Input: part model. Units: mm. Frame: model coordinates. A direction names the side the tool comes from. Coordinates: 2 decimals unless noted, no trailing zeros. Loops run counter-clockwise (first coordinate to the right, second up) from the corner with the lowest first, then second, coordinate; pieces in that order, holes last. Notation, with made-up numbers: (-15, 63) -> (34, 63) arc R10 ccw to (34, 69) -> close; hole circle Ø8 at (71, 85.25). An arc over 180 degrees is marked (long way). Put each result on its own line as item: value. Start each with the question number.
1) Cut plane A-A (z = 7.5). State how many separate pieces and enclosed holes the cut face has, plus the area to 3 significant figures.
2) Cut plane B-B (x = 19). Return the cut outline in (y, z), plus the area to 3 significant figures.
3) Material intervals for L1, parallel to Y at x = 24.5, z = 7.5; L2, parallel to Y at x = 5, z = 11; L3, parallel to Z at x = 19, y = 16.75, sorted ascending.
4) Cut plane D-D (x = 12.5). Return the cut outline in (y, z), plus the area to 3 significant figures.
5) Set-up query: faces 1 (the flat face through (27, -17, 7)), 2 (the flat face through (11, 14.1, 7.6)). Return all of +Z, -Z, +X, -X, +Y, -Y with unobstructed straight access to the full face (end or side cutting, diameter ignored); none if empty.
6) Contact query for flat-ended pins moving along their axis: P1, Ø1.5, axis at y = 10.5, z = 9.5, coming from the +X side; P2, Ø5.5, axis at x = 19, z = 7.5, coming from the -Y side. Output: stop coordinate, or through.
7) Pull-direction query (Z, two-part tool) for faces 3 (the conical face through (2.29, -18.75, 0.79)), 4 (the cylindrical face through (17.364, -17.128, 7.285)), 5 (the flat face through (13.6, 20.1, 14)), 6 (the flat face through (21, 15.1, 9)); classes: pulls with the +Z half, pulls with the -Z half, needs draft (parallel to the pull), parting line crosses it, or undercut.
Autodesk Inventor part; units mm, degrees
ref_plane "YZ Plane" through (0, 0, 0) normal (1, 0, 0) x (0, 1, 0)
ref_plane "XZ Plane" through (0, 0, 0) normal (0, 1, 0) x (-1, 0, 0)
ref_plane "XY Plane" through (0, 0, 0) normal (0, 0, 1) x (1, 0, 0)
sketch "スケッチ1" plane through (0, 0, 0) normal (0, 0, 1) x (1, 0, 0)
  line L0 (0, 21.1) -> (10, 21.1)
  line L1 (10, 21.1) -> (10, -21.1)
  line L2 (10, -21.1) -> (0, -21.1)
  line L3 (0, -21.1) -> (0, 21.1)
  line L4 (10, 21.1) -> (27, 21.1)
  line L5 (27, 21.1) -> (27, 15.1)
  line L6 (27, 15.1) -> (10, 15.1)
  line L7 (10, 15.1) -> (10, 21.1)
  line L8 (10, -21.1) -> (27, -21.1)
  line L9 (27, -21.1) -> (27, -15.1)
  line L10 (27, -15.1) -> (10, -15.1)
  line L11 (10, -15.1) -> (10, -21.1)
  point P0 (0, 0)
  point P1 (19, 15.1)
  point P2 (10, 15.1)
  dimension "d3" = 8
  dimension "d4" = 10
  dimension "d5" = 30.2
  dimension "d7" = 9
  dimension "d22" = 15.1
  dimension "d25" = 6
  dimension "d26" = 6
extrude "押し出し1" add sketch "スケッチ1" along normal blind 15
sketch "スケッチ2" plane through (0, 21.1, 0) normal (0, 1, 0) x (1, 0, 0)
  line L0 (27, -15) -> (0, -15)
  line L1 (27, 0) -> (27, -15)
  line L2 (27, 0) -> (10, 0)
  line L3 (10, 0) -> (10, -15)
  line L4 (27, -15) -> (10, -15)
  line L5 (27, 0) -> (27, -15)
  point P0 (19, -7.5)
  dimension "d10" = 8
  dimension "d11" = 7.5
hole "穴1" at (19, 21.1, 7.5) direction (0, -1, 0) diameter 3.3 depth 58
sketch "スケッチ3" plane through (0, 21.1, 0) normal (0, 1, 0) x (1, 0, 0)
  circle A0 centre (19, -7.5) radius 1.65
  circle A1 centre (19, -7.5) radius 2.2
  dimension "d19" = 4.4
extrude "押し出し2" cut sketch "スケッチ3" against normal blind 10 contours A0 | A1
fillet "フィレット2" radius 5 6 edges at (27, 18.1, 0) (27, -18.1, 0) (27, -18.1, 15) (27, 18.1, 15) (0, 21.1, 7.5) (0, -21.1, 7.5)
sketch "スケッチ7" plane through (0, 0, 0) normal (0, 0, -1) x (-1, 0, 0)
  circle A0 centre (-5, 0) radius 2.2
  point P0 (0, 0)
  dimension "d55" = 4.4
extrude "押し出し5" cut sketch "スケッチ7" against normal blind 21.25
sketch "スケッチ8" plane through (0, 0, 0) normal (0, 0, -1) x (-1, 0, 0)
  circle A0 centre (-5, 0) radius 2.2
  circle A1 centre (-5, 0) radius 1.75
  point P0 (0, 0)
  dimension "d65" = 3.5
extrude "押し出し6" add sketch "スケッチ8" against normal blind 10
chamfer "面取り8" distance 0.45 angle 45 1 edges at (6.75, 0, 10)
chamfer "面取り9" distance 2 angle 45 16 edges at (13.5, 21.1, 15) (1.4645, 19.6355, 15) (0, 0, 15) (1.4645, -19.6355, 15) (13.5, -21.1, 15) (25.5355, -21.1, 13.5355) (27, -21.1, 7.5) (25.5355, -21.1, 1.4645) (13.5, -21.1, 0) (1.4645, -19.6355, 0) (0, 0, 0) (1.4645, 19.6355, 0) (13.5, 21.1, 0) (25.5355, 21.1, 1.4645) (27, 21.1, 7.5) (25.5355, 21.1, 13.5355)
chamfer "面取り10" distance 2 angle 45 2 edges at (10, -15.1, 7.5) (10, 15.1, 7.5)
sketch "スケッチ9" plane through (5, -21.1, 2) normal (0, -1, 0) x (1, 0, 0)
  circle A0 centre (14, 5.5) radius 1.65
  point P0 (-5, -2)
hole "穴3" at (19, -21.1, 7.5) direction (0, 1, 0) diameter 6.5 depth 2
chamfer "面取り11" distance 0.5 angle 45 1 edges at (19, -21.1, 10.75)
properties part number "Print_Parts_I" material "PC/ABS プラスチック"
Results found:
1. separate pieces: 3
1. enclosed holes: 1
1. area: 553 mm2
2. outline: (-21.1, 2) -> (-19.1, 0) -> (-15.1, 0) -> (-15.1, 5.85) -> (-19.1, 5.85) -> (-19.1, 4.25) -> (-20.6, 4.25) -> (-21.1, 3.75) -> close; (-21.1, 11.25) -> (-20.6, 10.75) -> (-19.1, 10.75) -> (-19.1, 9.15) -> (-15.1, 9.15) -> (-15.1, 15) -> (-19.1, 15) -> (-21.1, 13) -> close; (15.1, 0) -> (19.1, 0) -> (21.1, 2) -> (21.1, 5.3) -> (15.1, 5.3) -> close; (15.1, 9.7) -> (21.1, 9.7) -> (21.1, 13) -> (19.1, 15) -> (15.1, 15) -> close
2. area: 119 mm2
3. L1: y = -21.1 to -15.1, 15.1 to 21.1
3. L2: y = -21.1 to -2.2, 2.2 to 21.1
3. L3: z = 0 to 5.3, 9.7 to 15
4. outline: (-21.1, 2) -> (-19.1, 0) -> (-15.1, 0) -> (-15.1, 15) -> (-19.1, 15) -> (-21.1, 13) -> close; (15.1, 0) -> (19.1, 0) -> (21.1, 2) -> (21.1, 13) -> (19.1, 15) -> (15.1, 15) -> close
4. area: 172 mm2
5. face 1: +Z, -Z, +X, +Y, -Y
5. face 2: +Z, -Z, +X
6. P1: stops at x = 10
6. P2: stops at y = -19.1
7. face 3: pulls with the -Z half
7. face 4: undercut
7. face 5: pulls with the +Z half
7. face 6: needs draft
